The model under review builds one solid part; all positions refer to its coordinate system, in mm. A direction names the side the tool comes from. Coordinates: 2 decimals unless noted, no trailing zeros. Write each loop counter-clockwise with the first axis right and the second up, starting at its lowest first coordinate (ties: lowest second). Pieces come first, ordered by that corner, then holes. Notation, with made-up numbers: (54, 66) - (69, 66) arc R11 ccw to (69, 82) - close; hole circle Ø5 at (42.5, -14.5). An arc over 180 degrees is marked (long way). Use one line per item in the form item = value. Start each with the question number.
```python
from build123d import *

# Parameters (mm, degrees)
SKETCH1_W           = 250
SKETCH1_H           = 20
BOSS_EXTRUDE1_DEPTH = 5
SKETCH2_W           = 250
SKETCH2_H           = 5
BOSS_EXTRUDE2_DEPTH = 80
BOSS_EXTRUDE3_DEPTH = 10
CUT_EXTRUDE2_DEPTH  = 10


with BuildPart() as part:
    # Sketch1 → Boss-Extrude1 (new body)
    with BuildSketch(Plane.XY):
        with Locations((125, 10)):
            Rectangle(SKETCH1_W, SKETCH1_H)
    extrude(amount=BOSS_EXTRUDE1_DEPTH)

    # Sketch2 → Boss-Extrude2 (add)
    with BuildSketch(Plane.XY.offset(5)):
        with Locations((125, 17.5)):
            Rectangle(SKETCH2_W, SKETCH2_H)
    extrude(amount=BOSS_EXTRUDE2_DEPTH)

    # Sketch4 → Boss-Extrude3 (add)
    with BuildSketch(Plane.XZ.offset(-15)):
        with BuildLine():
            Line((145, 31.244995812), (145, 65.71985119))
            ThreePointArc((145, 65.71985119), (150, 70.71985119), (155, 65.71985119))
            Line((155, 65.71985119), (155, 36.244995812))
            Line((155, 36.244995812), (214.286235525, 36.244995812))
            ThreePointArc((214.286235525, 36.244995812), (219.286235525, 31.244995812), (214.286235525, 26.244995812))
            Line((214.286235525, 26.244995812), (155, 26.244995812))
            Line((155, 26.244995812), (155, 5.178641746))
            ThreePointArc((155, 5.178641746), (150, 0.178641746), (145, 5.178641746))
            Line((145, 5.178641746), (145, 31.244995812))
        make_face()
    extrude(amount=BOSS_EXTRUDE3_DEPTH)

    # Sketch3 → Cut-Extrude2 (cut)
    with BuildSketch(Plane.XZ.offset(-15)):
        with BuildLine():
            Line((207.476121364, 69.762120736), (57.476121364, 21.762120736))
            ThreePointArc((57.476121364, 21.762120736), (54.059827752, 16.228833248), (59, 12))
            Line((59, 12), (189, 12))
            ThreePointArc((189, 12), (191.773500981, 12.839748528), (193.615384615, 15.076923077))
            Line((193.615384615, 15.076923077), (213.615384615, 63.076923077))
            ThreePointArc((213.615384615, 63.076923077), (212.682705424, 68.381964039), (207.476121364, 69.762120736))
        make_face()
        with BuildLine():
            Line((189.928273384, 53.647285584), (91.030505936, 22))
            Line((91.030505936, 22), (182.333333333, 22))
            ThreePointArc((182.333333333, 22), (185.106834314, 22.839748528), (186.948717949, 25.076923077))
            Line((186.948717949, 25.076923077), (196.067536635, 46.962087925))
            ThreePointArc((196.067536635, 46.962087925), (195.134857444, 52.267128886), (189.928273384, 53.647285584))
        make_face(mode=Mode.SUBTRACT)
    extrude(amount=-CUT_EXTRUDE2_DEPTH, mode=Mode.SUBTRACT)


solid = part.part
```
1. For P1, Ø2, axis at y = 5, z = 32.5, coming from the +X side; P2, Ø8, axis at x = 149.5, z = 17, coming from the +Y side; P3, Ø1, axis at x = 38, z = 26.5, coming from the -Y side; P4, Ø1.5, axis at y = 14, z = 72, coming from the +X side, all flat-tipped, find the tip position at first contact; note any pin that passes through.
2. Take a section at B-B (x = 150). State the section outline as (y, z) points.
3. For L1, parallel to Y at x = 115, z = 23.5; L2, parallel to X at y = 14.5, z = 8.5; L3, parallel to Y at x = 212, z = 32.5, list the stretches that pass through material, from the lowest coordinate up.
4. Take a section at C-C (x = 22). State the section outline as (y, z) points, plus the area to 3 significant figures.
5. The part is to be moulded in two halves that separate along X. For faces 4 (the cylindrical face through (54.046, 17.465, 16.327)), 5 (the flat face through (155, 10, 16)), 6 (the flat face through (123, 8, 5)), say which applies: released by +X, released by -X, zero draft, split by the parting line, or undercut.
6. For faces 1 (the flat face through (169, 5, 36)), 2 (the cylindrical face through (192, 17, 13)), 3 (the flat face through (195, 15, 31)), list the 3-axis set-ups (+Z, -Z, +X, -X, +Y, -Y) from which the entire face can be reached by the end or side of a thin tool; tool diameter is ignored.
7. Take a section at A-A (y = 10). State the section outline as (x, z) points (3 decimals), plus the area to 3 significant figures.
Returned:
q1.P1 = 219.28
q1.P2 = 15
q1.P3 = 15
q1.P4 = through
q2.outline = (0, 0) - (20, 0) - (20, 12) - (15, 12) - (15, 22) - (20, 22) - (20, 40.87) - (15, 40.87) - (15, 51.37) - (20, 51.37) - (20, 85) - (15, 85) - (15, 70.72) - (5, 70.72) - (5, 5) - (0, 5) - close
q3.L1 = 15 to 20
q3.L2 = 145 to 155
q3.L3 = 5 to 20
q4.outline = (0, 0) - (20, 0) - (20, 85) - (15, 85) - (15, 5) - (0, 5) - close
q4.area = 500 mm²
q5.face_4 = undercut
q5.face_5 = released by +X
q5.face_6 = zero draft
q6.face_1 = +Z, +X, -X, -Y
q6.face_2 = +Y, -Y
q6.face_3 = +Y
q7.outline = (0, 0) - (250, 0) - (250, 5) - (154.997, 5) arc R5 ccw to (155, 5.179) - (155, 26.245) - (214.286, 26.245) arc R5 ccw to (214.286, 36.245) - (155, 36.245) - (155, 65.72) arc R5 ccw to (145, 65.72) - (145, 5.179) arc R5 ccw to (145.003, 5) - (0, 5) - close
q7.area = 2,530 mm²
